```python
from build123d import *

# Parameters (mm, degrees)
F0_W     = 76.294
F0_H     = 76.294
F1_DEPTH = 0.5
F3_DEPTH = 0.5


with BuildPart() as f1:
    # F0 (on Front) → F1 (new body)
    with BuildSketch(Plane.XZ):
        with Locations((-38.147, 38.147)):
            Rectangle(F0_W, F0_H)
    extrude(amount=F1_DEPTH)

    # F2 (on face) → F3 (cut)
    with BuildSketch(Plane.XZ.offset(0.5)):
        Polygon((-74.574612, 4.273814), (-74.474379, 3.052396), (-3.142937, 3.052396), (-3.142937, 21.308729), (-21.963898, 21.308729), (-21.963898, 13.215715), (-8.412805, 13.215715), (-8.412805, 8.510474), (-34.19752, 8.510474), (-34.19752, 25.825759), (-3.331146, 25.825759), (-3.331146, 31.660259), (-45.301888, 31.660259), (-45.301888, 8.510474), (-73.533334, 8.510474), (-73.533334, 31.660259), (-53.394902, 31.660259), (-53.394902, 16.415277), (-58.476564, 16.415277), (-58.476564, 28.272485), (-66.757783, 28.272485), (-66.757783, 13.215715), (-49.066082, 13.215715), (-49.066082, 34.859821), (-73.721543, 34.859821), (-73.721543, 39.753273), (-45.490101, 39.753273), (-45.490101, 34.859821), (-3.331146, 34.859821), (-3.331146, 44.646721), (-73.721543, 44.646721), (-73.721543, 51.04585), (-3.331146, 51.04585), (-3.331146, 63.8441), (-12.741626, 63.8441), (-12.741626, 55.751089), (-24.410622, 55.751089), (-24.410622, 59.703492), (-17.446866, 59.703492), (-17.446866, 64.032309), (-30.997958, 64.032309), (-30.997958, 56.127511), (-73.721543, 56.127511), (-73.721543, 64.032309), (-66.757783, 64.032309), (-66.757783, 61.020955), (-35.89141, 61.020955), (-35.89141, 66.667251), (-3.331146, 66.667251), (-3.331146, 73.631003), (-73.721543, 73.631003), (-73.721543, 70.807859), (-39.090972, 70.807859), (-39.090972, 64.032309), (-45.866519, 64.032309), (-45.866519, 67.231879), (-73.721543, 67.231879), (-73.721543, 66.287316), (-47.128003, 66.287316), (-47.128003, 63.221127), (-38.352344, 63.221127), (-38.352344, 71.573861), (-72.714865, 71.573861), (-72.714865, 72.736897), (-4.307025, 72.736897), (-4.307025, 67.231879), (-37.083577, 67.231879), (-37.083577, 61.846625), (-65.948091, 61.846625), (-65.948091, 64.912818), (-74.829482, 64.912818), (-74.829482, 55.291314), (-29.893881, 55.291314), (-29.893881, 63.115396), (-18.474953, 63.115396), (-18.474953, 60.577855), (-25.558917, 60.577855), (-25.558917, 54.97412), (-11.496719, 54.97412), (-11.496719, 62.58674), (-4.307025, 62.58674), (-4.307025, 52.119389), (-74.935205, 52.119389), (-74.935205, 43.766655), (-4.307025, 43.766655), (-4.307025, 35.731114), (-44.590466, 35.731114), (-44.590466, 40.700462), (-74.935205, 40.700462), (-74.935205, 33.933688), (-50.194196, 33.933688), (-50.194196, 14.354197), (-65.555319, 14.354197), (-65.555319, 27.087314), (-59.586674, 27.087314), (-59.586674, 15.680563), (-52.291658, 15.680563), (-52.291658, 32.790691), (-74.935205, 32.790691), (-74.935205, 7.589729), (-44.068187, 7.589729), (-44.068187, 30.40323), (-4.307025, 30.40323), (-4.307025, 26.954677), (-35.89141, 26.954677), (-35.89141, 7.855003), (-6.929931, 7.855003), (-6.929931, 14.354197), (-20.856777, 14.354197), (-20.856777, 20.322846), (-4.277199, 20.322846), (-4.277199, 4.273814), align=None)
    extrude(amount=-F3_DEPTH, mode=Mode.SUBTRACT)


solid = f1.part
```
Input: part model. Units: mm. Frame: model coordinates. Give positions to 0.01 mm unless a question says otherwise; leave off trailing zeros. Order: outer loops, then holes, each group sorted by start corner. A loop starts at its lowest first (then second) coordinate and runs counter-clockwise, first axis right, second up.
1. Section A-A on z = 24. Give the number of separate pieces and of enclosed holes in the cut face, and give its area (3 significant figures).
Derived:
separate pieces: 8
enclosed holes: 0
area: 33.7 mm2
2. Section B-B on z = 69.5. Return the cut outline in (x, y).
Derived:
outline: (-76.29, -0.5) - (-39.09, -0.5) - (-39.09, 0) - (-76.29, 0) - close; (-38.35, -0.5) - (-4.31, -0.5) - (-4.31, 0) - (-38.35, 0) - close; (-3.33, -0.5) - (0, -0.5) - (0, 0) - (-3.33, 0) - close
3. Material intervals for L1, parallel to X at y = -0.25, z = 72; L2, parallel to X at y = -0.05, z = 58.5; L3, parallel to X at y = -0.3, z = 35, sorted ascending.
Derived:
L1: x = -76.29 to -73.72, -72.71 to -4.31, -3.33 to 0
L2: x = -76.29 to -74.83, -73.72 to -31, -29.89 to -25.56, -24.41 to -12.74, -11.5 to -4.31, -3.33 to 0
L3: x = -76.29 to -74.94, -73.72 to -45.49, -3.33 to 0
